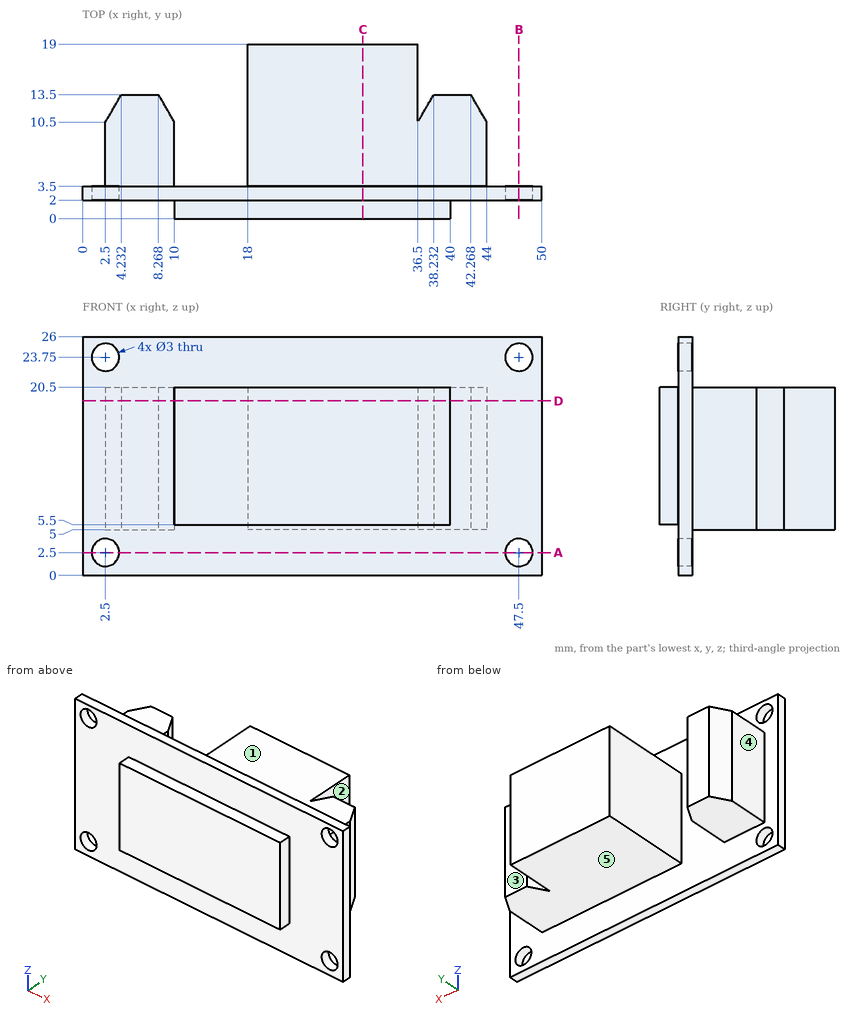
Could you check a few things on this drawing? It's one solid part, dimensions in mm from its lowest x, y, z. A direction names the side the tool comes from. Round coordinates to 2 decimals unless told otherwise and drop trailing zeros. Write each loop counter-clockwise with the first axis right and the second up, starting at its lowest first coordinate (ties: lowest second). Pieces come first, ordered by that corner, then holes. Notation, with made-up numbers: (47.25, 42) -> (63.25, 42) arc R16 ccw to (63.25, 54) -> close; hole circle Ø6 at (48, -1.75). An arc over 180 degrees is marked (long way). Use a Markdown table: item, result.
1. If we section it at A-A (z = 2.5): List the corners of the cut face in (x, y) for me.
Answer key:
| item | result |
|---|---|
| outline | (0, 2) -> (1, 2) -> (1, 3.5) -> (0, 3.5) -> close; (4, 2) -> (46, 2) -> (46, 3.5) -> (4, 3.5) -> close; (49, 2) -> (50, 2) -> (50, 3.5) -> (49, 3.5) -> close |
2. If we section it at B-B (x = 47.5): List the corners of the cut face in (y, z) for me.
Answer key:
| item | result |
|---|---|
| outline | (2, 0) -> (3.5, 0) -> (3.5, 1) -> (2, 1) -> close; (2, 4) -> (3.5, 4) -> (3.5, 22.25) -> (2, 22.25) -> close; (2, 25.25) -> (3.5, 25.25) -> (3.5, 26) -> (2, 26) -> close |
3. If we section it at C-C (x = 30.5): List the corners of the cut face in (y, z) for me, then the cut area to 3 significant figures.
Answer key:
| item | result |
|---|---|
| outline | (0, 5.5) -> (2, 5.5) -> (2, 0) -> (3.5, 0) -> (3.5, 5) -> (19, 5) -> (19, 20.5) -> (3.5, 20.5) -> (3.5, 26) -> (2, 26) -> (2, 20.5) -> (0, 20.5) -> close |
| area | 309 mm^2 |
4. Which directions (+Z, -Z, +X, -X, +Y, -Y) give clear straight access to the entire face, cutting with the end or side of a thin tool? Please do the marked faces 1, 2, 3, 4 and 5.
Answer key:
| item | result |
|---|---|
| face 1 | +Z, +X, -X, +Y |
| face 2 | +Z, -Z, +Y |
| face 3 | +Z, -Z, +X, +Y |
| face 4 | +Z, -Z, -X, +Y |
| face 5 | -Z, +X, -X, +Y |
5. If we section it at D-D (z = 19): List the corners of the cut face in (x, y) for me.
Answer key:
| item | result |
|---|---|
| outline | (0, 2) -> (10, 2) -> (10, 0) -> (40, 0) -> (40, 2) -> (50, 2) -> (50, 3.5) -> (44, 3.5) -> (44, 10.5) -> (42.27, 13.5) -> (38.23, 13.5) -> (36.5, 10.5) -> (36.5, 19) -> (18, 19) -> (18, 3.5) -> (10, 3.5) -> (10, 10.5) -> (8.27, 13.5) -> (4.23, 13.5) -> (2.5, 10.5) -> (2.5, 3.5) -> (0, 3.5) -> close |
6. For pin 1 Ø8.5 at (x, y) = (5.5, 10.5) entering from +Z; pin 2 Ø2 at (x, z) = (39.5, 10) entering from +Y; pin 3 Ø8 at (y, z) = (13.5, 21.5) entering from +X; pin 4 Ø5.5 at (y, z) = (5.5, 11) entering from -X, each with a flat end and sliding along its axis, tell me the tip position at first contact or that it passes through.
Answer key:
| item | result |
|---|---|
| pin 1 | stops at z = 20.5 |
| pin 2 | stops at y = 13.5 |
| pin 3 | stops at x = 44 |
| pin 4 | stops at x = 0 |
7. Please list where these lines run through material, in increasing order: probe 1 along Z at (x, y) = (2.5, 2.6); probe 2 along X at (y, z) = (3.25, 24.25); probe 3 along Z at (x, y) = (21, 4.5).
Answer key:
| item | result |
|---|---|
| probe 1 | z = 0 to 1, 4 to 22.25, 25.25 to 26 |
| probe 2 | x = 0 to 1.09, 3.91 to 46.09, 48.91 to 50 |
| probe 3 | z = 5 to 20.5 |
